The listing builds one solid part. Answer for the finished solid, in the listing's coordinates (mm). A direction names the side the tool comes from. Coordinates: 2 decimals unless noted, no trailing zeros. Order: outer loops, then holes, each group sorted by start corner. A loop starts at its lowest first (then second) coordinate and runs counter-clockwise, first axis right, second up. Notation, with made-up numbers: (57.5, 73) - (74.5, 73) arc R19 ccw to (74.5, 95) - close; hole circle Ø4 at (-5, 72). An arc over 180 degrees is marked (long way). Use a Markdown table: item, result. Add a question column.
Item 1: The part is cut by section A-A, the plane x = 5.25. Give the vertices of the cut face in (y, z).
Item 2: For faces 4 (the flat face through (6.2, 7, -17)), 5 (the flat face through (2.5, -9.3, 2.7)), 6 (the flat face through (0, -18, -6)), determine the directions among +Z, -Z, +X, -X, +Y, -Y from which every point of the face is accessible in a straight line to the end or side of a thin tool.
Item 3: Find the intervals of material crossed by line 1 along Y through (x, z) = (2.25, 0); line 2 along Y through (x, z) = (4, 0); line 3 along Y through (x, z) = (5, 0), in increasing order.
Item 4: The part is cut by section B-B, the plane x = 11.25. Give the vertices of the cut face in (y, z).
Item 5: The mould has two halves that part along Z. Classify faces 1 (the flat face through (6.5, 6, 17)), 2 (the conical face through (2.45, 11.47, 5.96)), 3 (the cylindrical face through (0.811, -21.565, -2.831)): released by +Z, released by -Z, zero draft, split by the parting line, or undercut.
Item 6: Flat-ended cylindrical pins translate along their axes: P1, Ø12, axis at y = 11.5, z = 15, coming from the +X side; P2, Ø5, axis at y = 13, z = 16.5, coming from the -X side; P3, Ø1.5, axis at x = 5, z = 9, coming from the +Y side; P4, Ø1, axis at x = 14, z = -8.5, coming from the +Y side. Find the tip coordinate at first contact, or state that the pin passes through.
from build123d import *
from build123d.topology import SkipClean

# Parameters (mm, degrees)
SKETCH3_R               = 9.5
BOSS_EXTRUDE1_DEPTH     = 16
CUT_EXTRUDE1_DEPTH      = 21.892582416
CUT_EXTRUDE1_DEPTH_BACK = 21.892582416
SHELL7_T                = -0.3
SKETCH8_R               = 10.705762979
CUT_EXTRUDE5_DEPTH      = 10


with BuildPart() as part:
    # Sketch3 → Boss-Extrude1 (new body)
    with BuildSketch(Plane.ZY):
        Circle(SKETCH3_R)
    extrude(amount=-BOSS_EXTRUDE1_DEPTH)

    # Sketch4 → Cut-Extrude1 (cut, two sides: drawn at the far end of the back side and taken through both)
    with BuildSketch(Plane.XY.offset(-CUT_EXTRUDE1_DEPTH_BACK)):
        Polygon((2.5, 9.5), (18.05891099, 17.267926144), (18.05891099, -17.267926144), (2.5, -9.5), (16, 0), align=None)
    extrude(amount=CUT_EXTRUDE1_DEPTH + CUT_EXTRUDE1_DEPTH_BACK, mode=Mode.SUBTRACT)

    # Shell7
    shell7_openings = [part.faces().sort_by_distance(p)[0] for p in [
        (0, 0, 0),
    ]]
    offset(amount=SHELL7_T, openings=shell7_openings, kind=Kind.INTERSECTION)

    # Sketch1 → Revolve1 (revolve)
    with SkipClean():  # the faces are left unmerged after this step: merging them gives an invalid solid
        with BuildSketch(Plane.XY, mode=Mode.PRIVATE) as revolve1_sk:
            Polygon((0, 18.75), (0, 21.75), (1.6, 21.75), (1.6, 19.05), (6.5, 19.05), (6.5, 17.65), (2.5, 12.5), (2.5, 9.5), (2.2, 9.5), (2.2, 12.602819589), (6.2, 17.752819589), (6.2, 18.75), align=None)
        revolve(revolve1_sk.sketch.rotate(Axis((0, 0, 0), (1, 0, 0)), 90), axis=Axis((0, 0, 0), (1, 0, 0)))

    # Sketch8 → Cut-Extrude5 (cut)
    with SkipClean():  # the faces are left unmerged after this step: merging them gives an invalid solid
        with BuildSketch(Plane.ZY.offset(-2.2)):
            Circle(SKETCH8_R)
        extrude(amount=CUT_EXTRUDE5_DEPTH, mode=Mode.SUBTRACT)


solid = part.part
Solution:
| question | item | result |
|---|---|---|
| 1 | outline | circle Ø38.1 at (0, 0); circle Ø33.06 at (0, 0); (-7.56, -5.75) arc R9.5 ccw to (7.56, -5.75) - (7.56, 5.75) arc R9.5 ccw to (-7.56, 5.75) - close; hole circle Ø37.5 at (0, 0); hole circle Ø32.08 at (0, 0); hole (-7.2, -5.73) arc R9.2 ccw to (7.2, -5.73) - (7.2, 5.73) arc R9.2 ccw to (-7.2, 5.73) - close |
| 2 | face 4 | -X |
| 2 | face 5 | +X |
| 2 | face 6 | +Z, -Z, -X, +Y, -Y |
| 3 | line 1 | y = -19.05 to -18.75, -12.67 to -9.2, 9.2 to 12.67, 18.75 to 19.05 |
| 3 | line 2 | y = -19.05 to -18.75, -14.92 to -14.43, -8.44 to -8.08, 8.08 to 8.44, 14.43 to 14.92, 18.75 to 19.05 |
| 3 | line 3 | y = -19.05 to -18.75, -16.21 to -15.72, -7.74 to -7.37, 7.37 to 7.74, 15.72 to 16.21, 18.75 to 19.05 |
| 4 | outline | (-3.34, -8.89) arc R9.5 ccw to (3.34, -8.89) - (3.34, 8.89) arc R9.5 ccw to (-3.34, 8.89) - close; hole (-2.98, -8.71) arc R9.2 ccw to (2.98, -8.71) - (2.98, 8.71) arc R9.2 ccw to (-2.98, 8.71) - close |
| 5 | face 1 | zero draft |
| 5 | face 2 | undercut |
| 5 | face 3 | split by the parting line |
| 6 | P1 | stops at x = 6.5 |
| 6 | P2 | stops at x = 0 |
| 6 | P3 | stops at y = 17.17 |
| 6 | P4 | stops at y = 1.76 |
